Geometry: see drawing. Coordinates: mm, zero at the bounding-box minimum. Coordinates: 2 decimals unless noted, no trailing zeros. Loops run counter-clockwise (first coordinate to the right, second up) from the corner with the lowest first, then second, coordinate; pieces in that order, holes last. Notation, with made-up numbers: (-7.5, 45) - (7.5, 45) arc R20 ccw to (7.5, 72) - close; hole circle Ø2 at (23, 22). An arc over 180 degrees is marked (long way). Use one line per item in the form item = value.
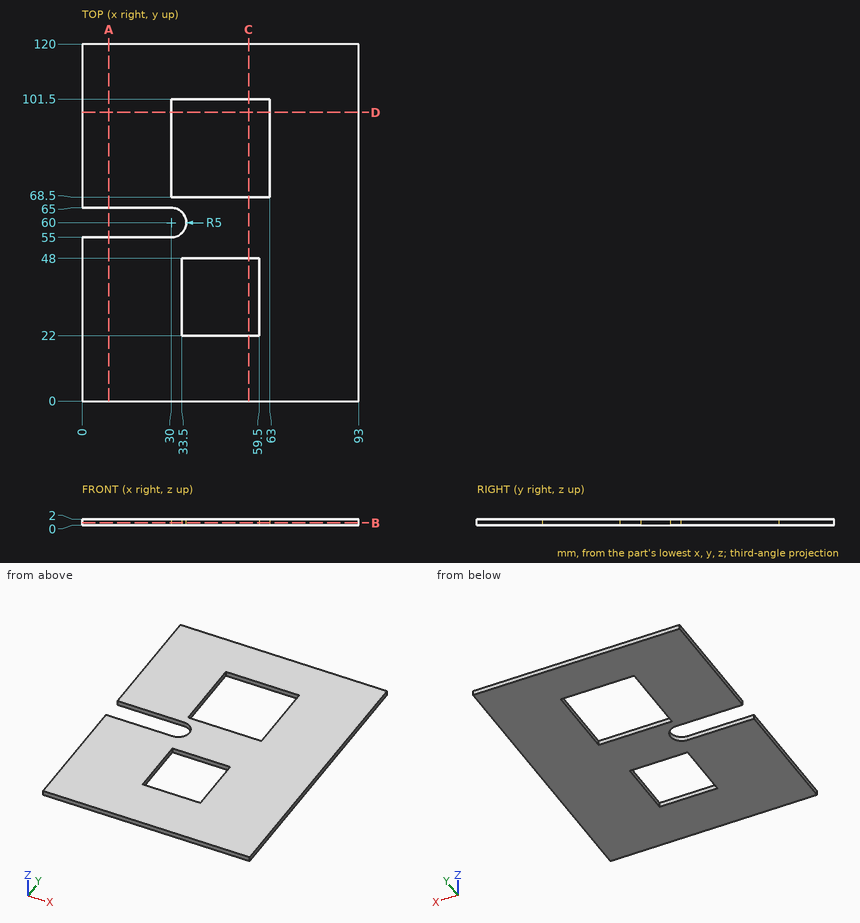
Q1. Cut plane C-C, the plane x = 56. Return loops of the section in (y, z).
Check values:
outline = (0, 0) - (22, 0) - (22, 2) - (0, 2) - close; (48, 0) - (68.5, 0) - (68.5, 2) - (48, 2) - close; (101.5, 0) - (120, 0) - (120, 2) - (101.5, 2) - close
Q2. Cut plane B-B, the plane z = 0.75. Return loops of the section in (x, y), then the cut area to 3 significant figures.
Check values:
outline = (0, 0) - (93, 0) - (93, 120) - (0, 120) - (0, 65) - (30, 65) arc R5 cw to (30, 55) - (0, 55) - close; hole (30, 68.5) - (63, 68.5) - (63, 101.5) - (30, 101.5) - close; hole (33.5, 22) - (59.5, 22) - (59.5, 48) - (33.5, 48) - close
area = 9,060 mm²
Q3. Cut plane A-A, the plane x = 9. Return loops of the section in (y, z), then the cut area to 3 significant figures.
Check values:
outline = (0, 0) - (55, 0) - (55, 2) - (0, 2) - close; (65, 0) - (120, 0) - (120, 2) - (65, 2) - close
area = 220 mm²
Q4. Cut plane D-D, the plane y = 97. Return loops of the section in (x, z), then the cut area to 3 significant figures.
Check values:
outline = (0, 0) - (30, 0) - (30, 2) - (0, 2) - close; (63, 0) - (93, 0) - (93, 2) - (63, 2) - close
area = 120 mm²
Q5. Ray query, line 1 along Y through (x, z) = (52.5, 1.25); line 2 along Y through (x, z) = (23, 1.55); line 3 along X through (y, z) = (46.5, 0.3). Return the intervals inside material, ascending. Write a range as [from, to].
Check values:
line_1 = [0, 22], [48, 68.5], [101.5, 120]
line_2 = [0, 55], [65, 120]
line_3 = [0, 33.5], [59.5, 93]
